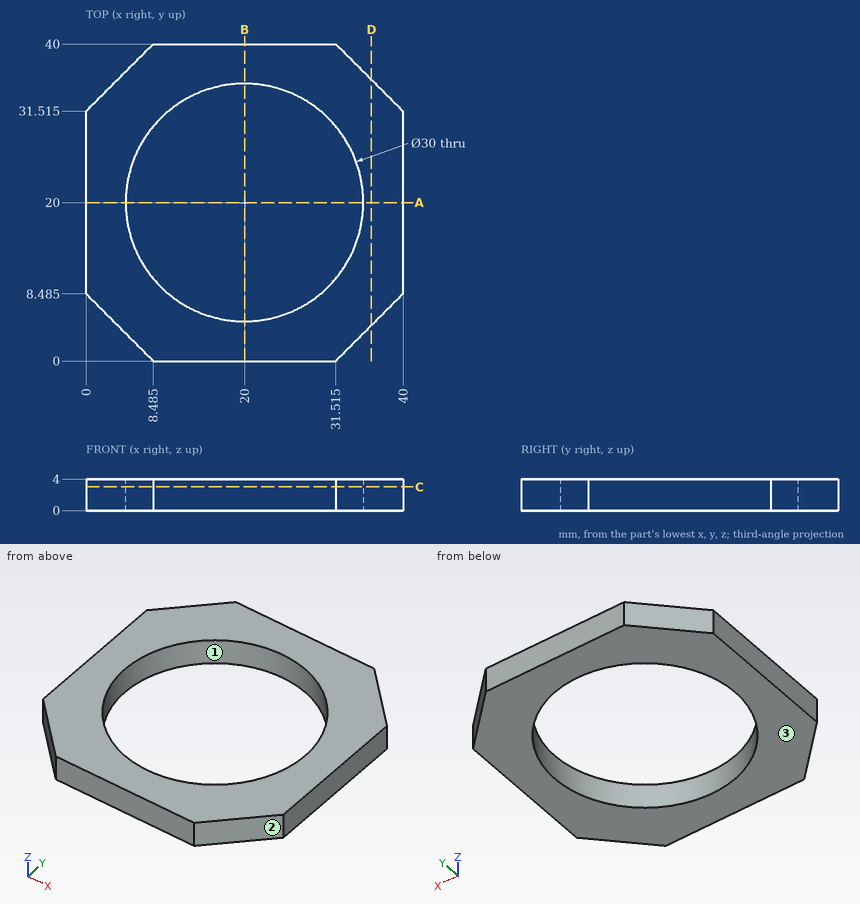
Print and shaded views of the part. All mm, measured from the part's lowest x, y and z. Coordinates: 2 decimals unless noted, no trailing zeros. Loops run counter-clockwise (first coordinate to the right, second up) from the corner with the lowest first, then second, coordinate; pieces in that order, holes last. Notation, with made-up numbers: (50.5, 77) -> (68.5, 77) arc R25 cw to (68.5, 112) -> close; hole circle Ø9 at (-24.75, 19). An arc over 180 degrees is marked (long way). Use one line per item in the form item = value. Start each with the question number.
(1) Pull direction X, two halves, no side cores. Call the marked faces 1, 2 and 3: pulls with the +X half, pulls with the -X half, needs draft (parallel to the pull), parting line crosses it, or undercut.
(2) Cut at A-A on y = 20. Give the cut face in (x, z), and give its area (3 significant figures).
(3) Probe probe 1 along Y at (x, z) = (20, 2.9); probe 2 along Y at (x, z) = (33.5, 3.5) (1 decimal); probe 3 along X at (y, z) = (27.5, 2). List the from-to ranges inside material, lowest first. Write a range as from..to.
(4) Cut at D-D on x = 36. Give the cut face in (y, z) (1 decimal), and give its area (3 significant figures).
(5) Cut at C-C on z = 3. Give the cut face in (x, y) (1 decimal), and give its area (3 significant figures).
Values:
q1.face_1 = undercut
q1.face_2 = pulls with the +X half
q1.face_3 = needs draft
q2.outline = (0, 0) -> (5, 0) -> (5, 4) -> (0, 4) -> close; (35, 0) -> (40, 0) -> (40, 4) -> (35, 4) -> close
q2.area = 40.0 mm2
q3.probe_1 = 0..5, 35..40
q3.probe_2 = 2..13.5, 26.5..38
q3.probe_3 = 0..7.01, 32.99..40
q4.outline = (4.5, 0) -> (35.5, 0) -> (35.5, 4) -> (4.5, 4) -> close
q4.area = 124 mm2
q5.outline = (0, 8.5) -> (8.5, 0) -> (31.5, 0) -> (40, 8.5) -> (40, 31.5) -> (31.5, 40) -> (8.5, 40) -> (0, 31.5) -> close; hole circle Ø30 at (20, 20)
q5.area = 749 mm2
